```python
from build123d import *

# Parameters (mm, degrees)
BOSS_EXTRUDE1_DEPTH                  = 12.5
F_20_0_20_DIAMETER_HOLE1_D           = 20
F_20_0_20_DIAMETER_HOLE1_CSINK_D     = 20.05
F_20_0_20_DIAMETER_HOLE1_CSINK_ANGLE = 90
CHAMFER2_SIZE                        = 2
CHAMFER3_SIZE                        = 2


with BuildPart() as part:
    # Sketch2 → Boss-Extrude1 (new, symmetric)
    with BuildSketch(Plane(origin=(0, 0, 0), x_dir=(0, 1, 0), z_dir=(0, 0, 1))):
        with BuildLine():
            Line((-140, -90), (140, -90))
            ThreePointArc((140, -90), (147.071067812, -87.071067812), (150, -80))
            Line((150, -80), (150, 80))
            ThreePointArc((150, 80), (147.071067812, 87.071067812), (140, 90))
            Line((140, 90), (-140, 90))
            ThreePointArc((-140, 90), (-147.071067812, 87.071067812), (-150, 80))
            Line((-150, 80), (-150, -80))
            ThreePointArc((-150, -80), (-147.071067812, -87.071067812), (-140, -90))
        make_face()
    extrude(amount=BOSS_EXTRUDE1_DEPTH, both=True)

    # Ø20.0 (20) Diameter Hole1 (through all)
    with Locations(Plane(origin=(-64.383356152, -125, 12.5), x_dir=(1, 0, 0), z_dir=(0, 0, 1))):
        with Locations((0, 0), (0, 125), (0, 250), (130, 250), (130, 125), (130, 0)):
            CounterSinkHole(F_20_0_20_DIAMETER_HOLE1_D / 2, F_20_0_20_DIAMETER_HOLE1_CSINK_D / 2, counter_sink_angle=F_20_0_20_DIAMETER_HOLE1_CSINK_ANGLE)

    # Chamfer2
    chamfer2_edges = [part.edges().sort_by_distance(p)[0] for p in [
        (87.071067812, 147.071067812, 12.5),
        (0, 150, 12.5),
        (-87.071067812, 147.071067812, 12.5),
        (-90, 0, 12.5),
        (-87.071067812, -147.071067812, 12.5),
        (0, -150, 12.5),
        (87.071067812, -147.071067812, 12.5),
        (90, 0, 12.5),
    ]]
    chamfer(chamfer2_edges, length=CHAMFER2_SIZE)

    # Chamfer3
    chamfer3_edges = [part.edges().sort_by_distance(p)[0] for p in [
        (0, 150, -12.5),
        (87.071067812, 147.071067812, -12.5),
        (90, 0, -12.5),
        (87.071067812, -147.071067812, -12.5),
        (75.616643848, -125, -12.5),
        (75.616643848, 0, -12.5),
        (75.616643848, 125, -12.5),
        (-54.383356152, 125, -12.5),
        (-54.383356152, 0, -12.5),
        (-54.383356152, -125, -12.5),
        (0, -150, -12.5),
        (-87.071067812, -147.071067812, -12.5),
        (-90, 0, -12.5),
        (-87.071067812, 147.071067812, -12.5),
    ]]
    chamfer(chamfer3_edges, length=CHAMFER3_SIZE)


solid = part.part
```
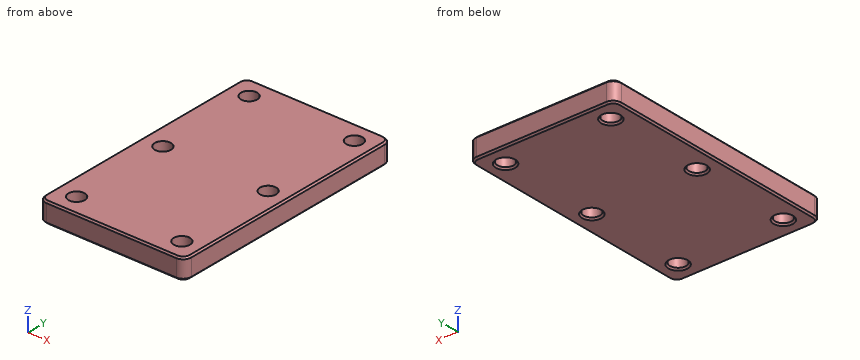
The model under review builds one solid part; all positions refer to its coordinate system, in mm. Round coordinates to 2 decimals unless told otherwise and drop trailing zeros. Loops run counter-clockwise (first coordinate to the right, second up) from the corner with the lowest first, then second, coordinate; pieces in that order, holes last.
1) Wall thickness on line 1 along X through (y, z) = (-125, 4): over which ranges is the line inside the solid? List them lowest first.
Values follow:
line 1: x = -90 to -74.38, -54.38 to 55.62, 75.62 to 90
2) Consider section C-C on y = 119. Give the number of separate pieces and of enclosed holes in the cut face, then the cut area to 3 significant figures.
Values follow:
separate pieces: 3
enclosed holes: 0
area: 3,680 mm2
3) Consider section B-B on y = 0. State the section outline as (x, z) points (3 decimals), then the cut area to 3 significant figures.
Values follow:
outline: (-90, -10.5) - (-88, -12.5) - (-76.383, -12.5) - (-74.383, -10.5) - (-74.383, 12.475) - (-74.408, 12.5) - (-88, 12.5) - (-90, 10.5) - close; (-54.383, -10.5) - (-52.383, -12.5) - (53.617, -12.5) - (55.617, -10.5) - (55.617, 12.475) - (55.592, 12.5) - (-54.358, 12.5) - (-54.383, 12.475) - close; (75.617, -10.5) - (77.617, -12.5) - (88, -12.5) - (90, -10.5) - (90, 10.5) - (88, 12.5) - (75.642, 12.5) - (75.617, 12.475) - close
area: 3,480 mm2
4) Consider section A-A on z = 2.75. State the section outline as (x, y) points.
Values follow:
outline: (-90, -140) arc R10 ccw to (-80, -150) - (80, -150) arc R10 ccw to (90, -140) - (90, 140) arc R10 ccw to (80, 150) - (-80, 150) arc R10 ccw to (-90, 140) - close; hole circle Ø20 at (-64.38, -125); hole circle Ø20 at (-64.38, 0); hole circle Ø20 at (-64.38, 125); hole circle Ø20 at (65.62, -125); hole circle Ø20 at (65.62, 0); hole circle Ø20 at (65.62, 125)
